```python
from build123d import *

# Parameters (mm, degrees)
SKETCH1_W           = 68
SKETCH1_H           = 39
BOSS_EXTRUDE1_DEPTH = 0.4


with BuildPart() as part:
    # Sketch1 → Boss-Extrude1 (new body)
    with BuildSketch(Plane(origin=(0, 0, 0), x_dir=(1, 0, 0), z_dir=(0, 1, 0))):
        with Locations((34, 19.5)):
            Rectangle(SKETCH1_W, SKETCH1_H)
        with BuildLine():
            ThreePointArc((20.292495584, 30.379077291), (17.832108181, 26.196960066), (16.614661349, 21.5))
            Line((16.614661349, 21.5), (29.171572875, 21.5))
            Line((29.171572875, 21.5), (20.292495584, 30.379077291))
        make_face(mode=Mode.SUBTRACT)
        with BuildLine():
            ThreePointArc((32, 36.885338651), (27.303039934, 35.667891819), (23.120922709, 33.207504416))
            Line((23.120922709, 33.207504416), (32, 24.328427125))
            Line((32, 24.328427125), (32, 36.885338651))
        make_face(mode=Mode.SUBTRACT)
        with BuildLine():
            ThreePointArc((44.879077291, 33.207504416), (40.696960066, 35.667891819), (36, 36.885338651))
            Line((36, 36.885338651), (36, 24.328427125))
            Line((36, 24.328427125), (44.879077291, 33.207504416))
        make_face(mode=Mode.SUBTRACT)
        with BuildLine():
            ThreePointArc((51.385338651, 21.5), (50.167891819, 26.196960066), (47.707504416, 30.379077291))
            Line((47.707504416, 30.379077291), (38.828427125, 21.5))
            Line((38.828427125, 21.5), (51.385338651, 21.5))
        make_face(mode=Mode.SUBTRACT)
        with BuildLine():
            ThreePointArc((47.707504416, 8.620922709), (50.167891819, 12.803039934), (51.385338651, 17.5))
            Line((51.385338651, 17.5), (38.828427125, 17.5))
            Line((38.828427125, 17.5), (47.707504416, 8.620922709))
        make_face(mode=Mode.SUBTRACT)
        with BuildLine():
            ThreePointArc((36, 2.114661349), (40.696960066, 3.332108181), (44.879077291, 5.792495584))
            Line((44.879077291, 5.792495584), (36, 14.671572875))
            Line((36, 14.671572875), (36, 2.114661349))
        make_face(mode=Mode.SUBTRACT)
        with BuildLine():
            ThreePointArc((23.120922709, 5.792495584), (27.303039934, 3.332108181), (32, 2.114661349))
            Line((32, 2.114661349), (32, 14.671572875))
            Line((32, 14.671572875), (23.120922709, 5.792495584))
        make_face(mode=Mode.SUBTRACT)
        with BuildLine():
            ThreePointArc((16.614661349, 17.5), (17.832108181, 12.803039934), (20.292495584, 8.620922709))
            Line((20.292495584, 8.620922709), (29.171572875, 17.5))
            Line((29.171572875, 17.5), (16.614661349, 17.5))
        make_face(mode=Mode.SUBTRACT)
    extrude(amount=BOSS_EXTRUDE1_DEPTH)


solid = part.part
```
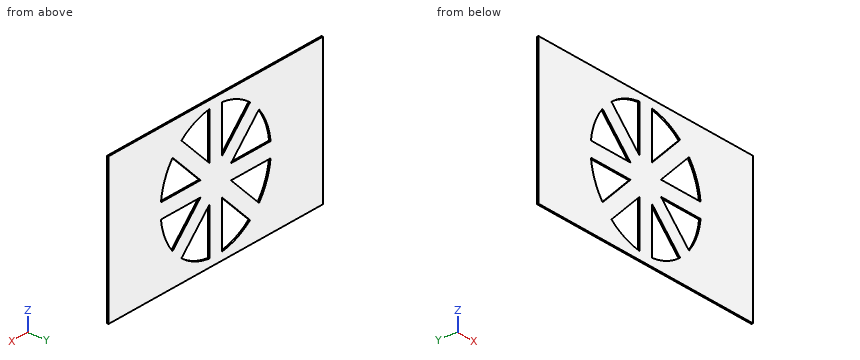
Geometry: final body of the model. Coordinates: model frame, mm. Give positions to 0.01 mm unless a question says otherwise; leave off trailing zeros. Write each loop counter-clockwise with the first axis right and the second up, starting at its lowest first coordinate (ties: lowest second). Pieces come first, ordered by that corner, then holes.
1. Pin query (flat end, axial travel): P1, Ø8, axis at x = 49, z = -21.5, coming from the -Y side. Return the tip coordinate at first contact, or that it passes through.
2. Section query B-B, the plane x = 39.5. Return loops of the section in (y, z), then the cut area to 3 significant figures.
3. Section query C-C, the plane y = 0.1. Count the separate pieces of the cut face and the enclosed holes in it, then the cut area to 3 significant figures.
4. Section query A-A, the plane z = -16.5. Return loops of the section in (x, y), then the cut area to 3 significant figures.
5. Line query: probe 1 along X at (y, z) = (0.3, -32); probe 2 along Z at (x, y) = (18.5, 0.3); probe 3 along X at (y, z) = (0.35, -9). Output: solid intervals per line, ascending.
6. Section query D-D, the plane z = -10. Return loops of the section in (x, y), then the cut area to 3 significant figures.
Computed:
1. P1: stops at y = 0
2. outline: (0, -39) - (0.4, -39) - (0.4, -36.11) - (0, -36.11) - close; (0, -27.83) - (0.4, -27.83) - (0.4, -22.17) - (0, -22.17) - close; (0, -21.5) - (0.4, -21.5) - (0.4, -17.5) - (0, -17.5) - close; (0, -16.83) - (0.4, -16.83) - (0.4, -11.17) - (0, -11.17) - close; (0, -2.89) - (0.4, -2.89) - (0.4, 0) - (0, 0) - close
2. area: 8.43 mm2
3. separate pieces: 1
3. enclosed holes: 8
3. area: 2,170 mm2
4. outline: (0, 0) - (16.76, 0) - (16.76, 0.4) - (0, 0.4) - close; (28.17, 0) - (39.83, 0) - (39.83, 0.4) - (28.17, 0.4) - close; (51.24, 0) - (68, 0) - (68, 0.4) - (51.24, 0.4) - close
4. area: 18.1 mm2
5. probe 1: x = 0 to 24.33, 32 to 36, 43.67 to 68
5. probe 2: z = -39 to -27.62, -21.5 to -17.5, -11.38 to 0
5. probe 3: x = 0 to 20, 20.67 to 26.33, 32 to 36, 41.67 to 47.33, 48 to 68
6. outline: (0, 0) - (19.3, 0) - (19.3, 0.4) - (0, 0.4) - close; (21.67, 0) - (27.33, 0) - (27.33, 0.4) - (21.67, 0.4) - close; (32, 0) - (36, 0) - (36, 0.4) - (32, 0.4) - close; (40.67, 0) - (46.33, 0) - (46.33, 0.4) - (40.67, 0.4) - close; (48.7, 0) - (68, 0) - (68, 0.4) - (48.7, 0.4) - close
6. area: 21.6 mm2
